Build history of the part. All positions in model axes, mm. A direction names the side the tool comes from. Coordinates: 2 decimals unless noted, no trailing zeros. Loops run counter-clockwise (first coordinate to the right, second up) from the corner with the lowest first, then second, coordinate; pieces in that order, holes last. Notation, with made-up numbers: (14, -20.75) - (64, -20.75) arc R12 ccw to (64, -5.75) - close; hole circle Ø2 at (-39.5, -12.75). An arc over 180 degrees is marked (long way). One line per item, written item: value.
```python
from build123d import *

# Parameters (mm, degrees)
SKETCH1_R           = 11.7
BOSS_EXTRUDE1_DEPTH = 25.4
BOSS_EXTRUDE1_DRAFT = -5
SKETCH2_R           = 3.175
CUT_EXTRUDE1_DEPTH  = 31.314023158
SKETCH9_R           = 7.35
CUT_EXTRUDE3_DEPTH  = 12.7
SKETCH14_R          = 1.75
CUT_EXTRUDE5_DEPTH  = 7.62


with BuildPart() as part:
    # Sketch1 → Boss-Extrude1 (with draft: the straight prism first)
    with BuildSketch(Plane(origin=(0, 0, 0), x_dir=(1, 0, 0), z_dir=(0, 1, 0))):
        Circle(SKETCH1_R)
    extrude(amount=-BOSS_EXTRUDE1_DEPTH)
    # Boss-Extrude1: the draft: its side faces are tilted about the plane it starts from
    boss_extrude1_sides = [part.faces().sort_by_distance(p)[0] for p in [
        (-11.7, -12.7, 0),
    ]]
    draft(boss_extrude1_sides, Plane(origin=(0, 0, 0), x_dir=(1, 0, 0), z_dir=(0, 1, 0)), BOSS_EXTRUDE1_DRAFT)

    # Sketch2 → Cut-Extrude1 (cut, through all)
    with BuildSketch(Plane(origin=(0, 0, 0), x_dir=(1, 0, 0), z_dir=(0, 1, 0))):
        with Locations(Location((0, 0, 0), (0, 0, 270))):
            Circle(SKETCH2_R)
    extrude(amount=-CUT_EXTRUDE1_DEPTH, mode=Mode.SUBTRACT)

    # Sketch9 → Cut-Extrude3 (cut)
    with BuildSketch(Plane(origin=(0, 0, 0), x_dir=(1, 0, 0), z_dir=(0, 1, 0))):
        with Locations(Location((0, 0, 0), (0, 0, 270))):
            Circle(SKETCH9_R)
    extrude(amount=-CUT_EXTRUDE3_DEPTH, mode=Mode.SUBTRACT)

    # Sketch14 → Cut-Extrude5 (cut)
    with BuildSketch(Plane.XZ.offset(25.4)):
        with Locations(Location((-5.826393973, 0, 0), (0, 0, 270))):
            Circle(SKETCH14_R)
        with Locations(Location((0, 5.826393973, 0), (0, 0, 270))):
            Circle(SKETCH14_R)
        with Locations(Location((5.826393973, 0, 0), (0, 0, 270))):
            Circle(SKETCH14_R)
        with Locations(Location((0, -5.826393973, 0), (0, 0, 270))):
            Circle(SKETCH14_R)
    extrude(amount=-CUT_EXTRUDE5_DEPTH, mode=Mode.SUBTRACT)


solid = part.part
```
Item 1: Probe probe 1 along Z at (x, y) = (-0.25, -20); probe 2 along X at (y, z) = (-22.25, 0) (3 decimals); probe 3 along X at (y, z) = (-8.75, -1.5). List the from-to ranges inside material, lowest first. Write a range as from..to.
Check result:
probe 1: z = -9.95..-7.56, -4.09..-3.17, 3.17..4.09, 7.56..9.95
probe 2: x = -9.753..-7.576, -4.076..-3.175, 3.175..4.076, 7.576..9.753
probe 3: x = -10.83..-7.2, 7.2..10.83
Item 2: Pull direction Z, two halves, no side cores. Call faces 1 (the face through (2, -25.4, 4)), 2 (the face through (-7.175, -6.261, -1.593)), 3 (the face through (0.077, -21.643, 7.575)), 4 (the face through (5.701, -12.522, -8.942)): released by +Z, released by -Z, zero draft, split by the parting line, or undercut.
Check result:
face 1: zero draft
face 2: undercut
face 3: undercut
face 4: split by the parting line
Item 3: Cut at B-B, the plane z = 0. Write the cut outline in (x, y) (3 decimals), then the cut area to 3 significant figures.
Check result:
outline: (-11.7, 0) - (-9.478, -25.4) - (-7.576, -25.4) - (-7.576, -17.78) - (-4.076, -17.78) - (-4.076, -25.4) - (-3.175, -25.4) - (-3.175, -12.7) - (-7.35, -12.7) - (-7.35, 0) - close; (3.175, -25.4) - (4.076, -25.4) - (4.076, -17.78) - (7.576, -17.78) - (7.576, -25.4) - (9.478, -25.4) - (11.7, 0) - (7.35, 0) - (7.35, -12.7) - (3.175, -12.7) - close
area: 217 mm^2
Item 4: Tool access for faces 5 (the face through (8, 0, 0)), 6 (the face through (-6, -17.78, 0)), 7 (the face through (-2, -12.7, 3)): list every direction of +Z, -Z, +X, -X, +Y, -Y with a clear straight run to the whole face (end or side of a thin tool).
Check result:
face 5: +Z, -Z, +X, -X, +Y
face 6: -Y
face 7: +Y
Item 5: Cut at D-D, the plane y = -4.25. Write the cut outline in (x, z), then the cut area to 3 significant figures.
Check result:
outline: circle Ø22.66 at (0, 0); hole circle Ø14.7 at (0, 0)
area: 233 mm^2
Item 6: Drop flat-ended pins along their axis: P1, Ø7.5, axis at x = 0, z = 0, coming from the +Y side; P2, Ø1, axis at x = 3, y = -7, coming from the -Z side; P3, Ø4, axis at y = -17.5, z = 8.5, coming from the +X side. Give the stop position or say it passes through.
Check result:
P1: stops at y = -12.7
P2: stops at z = -10.81
P3: stops at x = 7.84
Item 7: Cut at C-C, the plane y = -21. Write the cut outline in (x, z) (3 decimals).
Check result:
outline: circle Ø19.725 at (0, 0); hole circle Ø3.5 at (-5.826, 0); hole circle Ø6.35 at (0, 0); hole circle Ø3.5 at (0, -5.826); hole circle Ø3.5 at (0, 5.826); hole circle Ø3.5 at (5.826, 0)
Item 8: Cut at A-A, the plane x = 0. Write the cut outline in (y, z) (3 decimals).
Check result:
outline: (-25.4, -9.478) - (0, -11.7) - (0, -7.35) - (-12.7, -7.35) - (-12.7, -3.175) - (-25.4, -3.175) - (-25.4, -4.076) - (-17.78, -4.076) - (-17.78, -7.576) - (-25.4, -7.576) - close; (-25.4, 3.175) - (-12.7, 3.175) - (-12.7, 7.35) - (0, 7.35) - (0, 11.7) - (-25.4, 9.478) - (-25.4, 7.576) - (-17.78, 7.576) - (-17.78, 4.076) - (-25.4, 4.076) - close
